The model under review builds one solid part; all positions refer to its coordinate system, in mm. A direction names the side the tool comes from. Coordinates: 2 decimals unless noted, no trailing zeros. Order: outer loops, then holes, each group sorted by start corner. A loop starts at its lowest first (then second) coordinate and runs counter-clockwise, first axis right, second up. Notation, with made-up numbers: M -8.75,56.5 L 10.25,56.5 A22 ccw 10.25,81.5 Z; hole C 48,78 d8. An arc over 180 degrees is marked long. One line per item, written item: value.
```python
from build123d import *

# Parameters (mm, degrees)
SKETCH2_R          = 6.35
CUT_EXTRUDE1_DEPTH = 657.861735142


with BuildPart() as part:
    # Sketch1 → Revolve1 (revolve)
    with BuildSketch(Plane.XY, mode=Mode.PRIVATE) as revolve1_sk:
        Polygon((101.6, -36.990823201), (101.6, 318.609176799), (161.358198728, 318.609176799), (161.358198728, 324.959176799), (101.6, 324.959176799), (0, 324.959176799), (0, 318.609176799), (0, -290.990823201), (101.6, -290.990823201), (101.6, -43.340823201), (161.358198728, -43.340823201), (161.358198728, -36.990823201), align=None)
        Polygon((101.6, 324.959176799), (0, 324.959176799), (0, 318.609176799), (0, -290.990823201), (101.6, -290.990823201), (101.6, -43.340823201), (161.358198728, -43.340823201), (161.358198728, -36.990823201), (101.6, -36.990823201), (101.6, 318.609176799), (161.358198728, 318.609176799), (161.358198728, 324.959176799), align=None)
    revolve(revolve1_sk.sketch.rotate(Axis((0, 318.609176799, 0), (0, -1, 0)), 180), axis=Axis((0, 318.609176799, 0), (0, -1, 0)))

    # Sketch2 → Cut-Extrude1 (cut, through all)
    with BuildSketch(Plane(origin=(0, 324.959176799, 0), x_dir=(1, 0, 0), z_dir=(0, 1, 0))):
        with Locations(Location((0, 139.7, 0), (0, 0, 180))):
            Circle(SKETCH2_R)
        with Locations(Location((120.983748909, 69.85, 0), (0, 0, 180))):
            Circle(SKETCH2_R)
        with Locations(Location((120.983748909, -69.85, 0), (0, 0, 180))):
            Circle(SKETCH2_R)
        with Locations(Location((0, -139.7, 0), (0, 0, 180))):
            Circle(SKETCH2_R)
        with Locations(Location((-120.983748909, -69.85, 0), (0, 0, 180))):
            Circle(SKETCH2_R)
        with Locations(Location((-120.983748909, 69.85, 0), (0, 0, 180))):
            Circle(SKETCH2_R)
    extrude(amount=-CUT_EXTRUDE1_DEPTH, mode=Mode.SUBTRACT)


solid = part.part
```
(1) Insertion check: pin 1 Ø14.5 at (x, z) = (0, 139.7) entering from -Y; pin 2 Ø6 at (x, y) = (28.5, -41) entering from +Z; pin 3 Ø2 at (x, y) = (-37.5, -16) entering from -Z; pin 4 Ø14.5 at (x, z) = (-120.98, -69.85) entering from +Y. Each pin has a flat end and moves straight along its axis. Give the tip position at first contact, or say it passes through.
Geometry results:
pin 1: stops at y = -43.34
pin 2: stops at z = 159.33
pin 3: stops at z = -94.82
pin 4: stops at y = 324.96
(2) Tool access review of faces 1 (the cylindrical face through (21.006, -40.121, -159.985)), 2 (the cylindrical face through (-46.88, 143.3, 90.14)): name each direction out of +Z, -Z, +X, -X, +Y, -Y from which nothing blocks a thin tool from reaching the whole face with its end or side.
Geometry results:
face 1: +Y, -Y
face 2: none
(3) We need section D-D, the plane x = 136.5. State the section outline as (y, z) points, plus the area to 3 significant figures.
Geometry results:
outline: M -43.34,-86.05 L -36.99,-86.05 L -36.99,86.05 L -43.34,86.05 Z; M 318.61,-86.05 L 324.96,-86.05 L 324.96,86.05 L 318.61,86.05 Z
area: 2,190 mm2
(4) We need section C-C, the plane z = -139.7. State the section outline as (x, y) points, plus the area to 3 significant figures.
Geometry results:
outline: M -80.75,-43.34 L -6.35,-43.34 L -6.35,-36.99 L -80.75,-36.99 Z; M -80.75,318.61 L -6.35,318.61 L -6.35,324.96 L -80.75,324.96 Z; M 6.35,-43.34 L 80.75,-43.34 L 80.75,-36.99 L 6.35,-36.99 Z; M 6.35,318.61 L 80.75,318.61 L 80.75,324.96 L 6.35,324.96 Z
area: 1,890 mm2
(5) Mouldability with a two-part tool opening along X and no side actions: class faces 3 (the cylindrical face through (-46.88, -165.43, 90.14)), 4 (the flat face through (105, 318.609, -2)), 5 (the cylindrical face through (127.328, -40.121, -69.571)) as +X half, -X half, draft (parallel to the pull), parting line (faces both ways), or undercut.
Geometry results:
face 3: parting line
face 4: draft
face 5: undercut
(6) We need section B-B, the plane z = 0. State the section outline as (x, y) points, plus the area to 3 significant figures.
Geometry results:
outline: M -161.36,-43.34 L -101.6,-43.34 L -101.6,-290.99 L 101.6,-290.99 L 101.6,-43.34 L 161.36,-43.34 L 161.36,-36.99 L 101.6,-36.99 L 101.6,318.61 L 161.36,318.61 L 161.36,324.96 L -161.36,324.96 L -161.36,318.61 L -101.6,318.61 L -101.6,-36.99 L -161.36,-36.99 Z
area: 127,000 mm2
(7) We need section A-A, the plane x = 0. Count the separate pieces of the cut face and the enclosed holes in it, plus the area to 3 significant figures.
Geometry results:
separate pieces: 5
enclosed holes: 0
area: 126,000 mm2
(8) For L1, parallel to Z at x = 0, y = -40; L2, parallel to Y at x = -13.5, z = 132; L3, parallel to X at y = 321, z = 69, list the stretches that pass through material, from the lowest coordinate up.
Geometry results:
L1: z = -161.36 to -146.05, -133.35 to 133.35, 146.05 to 161.36
L2: y = -43.34 to -36.99, 318.61 to 324.96
L3: x = -145.86 to -127.28, -114.69 to 114.69, 127.28 to 145.86
